The model under review builds one solid part; all positions refer to its coordinate system, in mm. Face numbers are marked on the shaded views. A direction names the side the tool comes from. Coordinates: 2 decimals unless noted, no trailing zeros. Order: outer loops, then holes, each group sorted by start corner. A loop starts at its lowest first (then second) coordinate and runs counter-clockwise, first axis right, second up. Notation, with made-up numbers: M 31.25,83.25 L 90.25,83.25 A15 cw 90.25,106.25 Z; hole C -13,73.25 d6. An arc over 180 degrees is marked long. Answer as CSV lines item,"result". Start each with the question number.
Q1. Consider section B-B on z = -31.15. Write out the cut boundary in (x, y).
Q2. Machinability: for the marked faces 1, 2, 3 and 4, which of the approach directions +Z, -Z, +X, -X, +Y, -Y give a long, thin tool a straight path to every point of the face, cutting with its end or side? Answer none if there is none.
Q3. Wall thickness on L1, parallel to X at y = 880.5, z = -16; L2, parallel to X at y = 905, z = -31; L3, parallel to Z at x = 112, y = 921: over which ranges is each line inside the solid? List them lowest first. Write a range as [from, to].
Q4. Consider section D-D on z = -39.5. Write out the cut boundary in (x, y), and give its area (3 significant figures).
Q5. Consider section C-C on x = 164.5. Write out the cut boundary in (y, z).
Q6. For P1, Ø4, axis at x = 54.5, z = -32, coming from the +Y side; P2, Ø6.5, axis at y = 903.5, z = -31, coming from the +X side; P3, Ø10, axis at x = 93, z = -19.5, coming from the +Y side, all flat-tipped, find the tip position at first contact; note any pin that passes through.
Q7. Consider section A-A on y = 903.5. Write out the cut boundary in (x, z), and give its area (3 significant figures).
from build123d import *

# Parameters (mm, degrees)
SKETCH1_W                = 150
SKETCH1_H                = 10
BOSS_EXTRUDE1_DEPTH      = 55
SKETCH2_W                = 150
SKETCH2_H                = 10
BOSS_EXTRUDE2_DEPTH      = 45
BOSS_EXTRUDE2_DEPTH_BACK = 55
SKETCH3_W                = 45
SKETCH3_H                = 8
BOSS_EXTRUDE3_DEPTH      = 42
SKETCH4_W                = 56.520568853
SKETCH4_H                = 45
CUT_EXTRUDE1_DEPTH       = 56
SKETCH5_R                = 11.5
CUT_EXTRUDE2_DEPTH       = 80


with BuildPart() as part:
    # Sketch1 → Boss-Extrude1 (new body)
    with BuildSketch(Plane.XY):
        with Locations((112.750906932, 878.250348045)):
            Rectangle(SKETCH1_W, SKETCH1_H)
    extrude(amount=-BOSS_EXTRUDE1_DEPTH)

    # Sketch2 → Boss-Extrude2 (add, two sides)
    with BuildSketch(Plane(origin=(0, 883.250348045, 0), x_dir=(1, 0, 0), z_dir=(0, 1, 0))) as boss_extrude2_sk:
        with Locations((112.750906932, 5)):
            Rectangle(SKETCH2_W, SKETCH2_H)
    extrude(amount=BOSS_EXTRUDE2_DEPTH)
    extrude(boss_extrude2_sk.sketch, amount=-BOSS_EXTRUDE2_DEPTH_BACK)

    # Sketch3 → Boss-Extrude3 (add)
    with BuildSketch(Plane(origin=(0, 0, -10), x_dir=(-1, 0, 0), z_dir=(0, 0, -1))):
        with Locations((-112.750906932, 903.250348045)):
            Rectangle(SKETCH3_W, SKETCH3_H)
    extrude(amount=BOSS_EXTRUDE3_DEPTH)

    # Sketch4 → Cut-Extrude1 (cut, through all)
    with BuildSketch(Plane(origin=(0, 883.250348045, 0), x_dir=(1, 0, 0), z_dir=(0, 1, 0))):
        with Locations((113.076467001, 32.5)):
            Rectangle(SKETCH4_W, SKETCH4_H)
    extrude(amount=-CUT_EXTRUDE1_DEPTH, mode=Mode.SUBTRACT)

    # Sketch5 → Cut-Extrude2 (cut, through all)
    with BuildSketch(Plane(origin=(0, 907.250348045, 0), x_dir=(1, 0, 0), z_dir=(0, 1, 0))):
        with Locations((112.600906932, 31.15)):
            Circle(SKETCH5_R)
    extrude(amount=-CUT_EXTRUDE2_DEPTH, mode=Mode.SUBTRACT)


solid = part.part
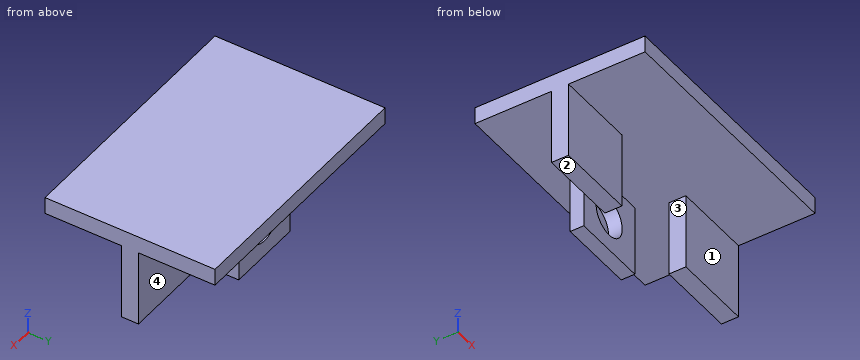
Evaluation:
1,outline,"M 37.75,873.25 L 84.82,873.25 L 84.82,883.25 L 37.75,883.25 Z; M 90.25,899.25 L 101.1,899.25 L 101.1,907.25 L 90.25,907.25 Z; M 124.1,899.25 L 135.25,899.25 L 135.25,907.25 L 124.1,907.25 Z; M 141.34,873.25 L 187.75,873.25 L 187.75,883.25 L 141.34,883.25 Z"
2,face 1,"-Z, +X, -X, -Y"
2,face 2,"-Z, +X, -X, +Y, -Y"
2,face 3,"-Z, +Y, -Y"
2,face 4,"-Z, +X, -X, +Y"
3,L1,"x = [37.75, 84.82], [141.34, 187.75]"
3,L2,"x = [90.25, 101.1], [124.1, 135.25]"
3,L3,"z = [-10, 0]"
4,outline,"M 37.75,873.25 L 84.82,873.25 L 84.82,883.25 L 37.75,883.25 Z; M 90.25,899.25 L 104.69,899.25 L 104.69,907.25 L 90.25,907.25 Z; M 120.51,899.25 L 135.25,899.25 L 135.25,907.25 L 120.51,907.25 Z; M 141.34,873.25 L 187.75,873.25 L 187.75,883.25 L 141.34,883.25 Z"
4,area,"1,170 mm²"
5,outline,"M 828.25,-10 L 873.25,-10 L 873.25,-55 L 883.25,-55 L 883.25,-10 L 928.25,-10 L 928.25,0 L 828.25,0 Z"
6,P1,"stops at y = 883.25"
6,P2,"stops at x = 135.25"
6,P3,"stops at y = 907.25"
7,outline,"M 37.75,-10 L 90.25,-10 L 90.25,-52 L 135.25,-52 L 135.25,-10 L 187.75,-10 L 187.75,0 L 37.75,0 Z; hole C 112.6,-31.15 d23"
7,area,"2,970 mm²"
